Read the model definition and answer for the solid it produces. Units are mm, in the model's axes. Face numbers are marked on the shaded views. A direction names the side the tool comes from. Give positions to 0.01 mm unless a question says otherwise; leave off trailing zeros. Loops run counter-clockwise (first coordinate to the right, second up) from the corner with the lowest first, then second, coordinate; pieces in that order, holes last. Notation, with made-up numbers: (6.5, 49) - (20.5, 49) arc R30 ccw to (20.5, 88) - close; hole circle Ø9 at (55, -20). An arc over 180 degrees is marked (long way). Write each question's results on one line, items separated by ' | '. Start each with the question number.
Q1. The part is cut by section A-A, the plane z = 1. Write down the section's boundary in (x, y).
Q2. The part is cut by section C-C, the plane y = 81.5. Write down the section's boundary in (x, z), plus the area to 3 significant figures.
Q3. Given pin 1 (1.5 mm diameter, centred on x = 3.5, z = 1.5, fed in from -Y); pin 2 (2.5 mm diameter, centred on x = -5, z = 6, fed in from -Y); pin 3 (2.5 mm diameter, centred on x = 0, y = 100, fed in from -Z); pin 4 (2 mm diameter, centred on y = 93.5, z = 4.5, fed in from -X), each flat-ended and moving along its own axis, determine where each tip first touches the part or whether it passes through.
Q4. The part is cut by section D-D, the plane z = 6. State how many separate pieces and enclosed holes the cut face has, plus the area to 3 significant figures.
Q5. For the marked faces 4, 5, 6 and 7, determine the directions among +Z, -Z, +X, -X, +Y, -Y from which every point of the face is accessible in a straight line to the end or side of a thin tool.
Q6. Find the intervals of material crossed by line 1 (Y direction, x = 0, z = 1.6); line 2 (X direction, y = 55.5, z = 6); line 3 (Y direction, x = 11.5, z = 8.5), in increasing order. Write a range as from..to.
Q7. Determine the mould class of the marked faces 1, 2 and 3 for opening direction Y: +Y half, -Y half, draft (parallel to the pull), parting line (faces both ways), or undercut.
Q8. The part is cut by section B-B, the plane x = -8. Write down the section's boundary in (y, z).
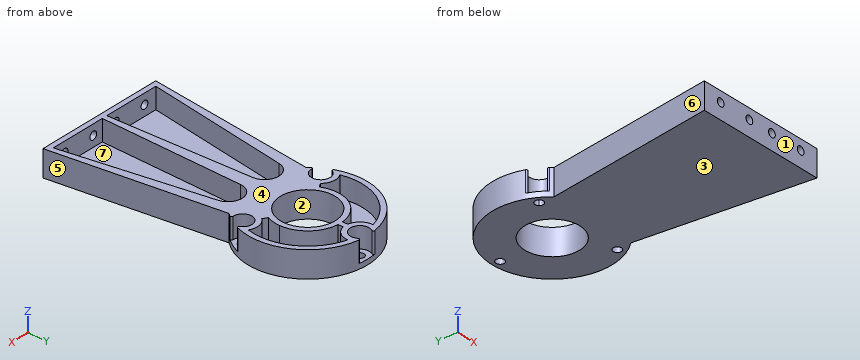
```python
from build123d import *

# Parameters (mm, degrees)
SKETCH_1_R          = 10.5
EXTRUDE_1_DEPTH     = 10
CUT_EXTRUDE_2_DEPTH = 8
SKETCH_3_R          = 1.5
CUT_EXTRUDE_3_DEPTH = 97.81941954
EXTRUDE_START       = -10
SKETCH_4_R          = 1.6
EXTRUDE_3_DEPTH     = 10
CUT_EXTRUDE_START   = -10
SKETCH_5_R          = 1.6
CUT_EXTRUDE_4_DEPTH = 10
CUT_EXTRUDE_START_2 = -8
SKETCH_6_R          = 1.6
CUT_EXTRUDE_5_DEPTH = 8
FILLET_1_R          = 0.5


with BuildPart() as part:
    # 草图1 → 凸台-拉伸1 (new body)
    with BuildSketch(Plane.XY):
        with BuildLine():
            Line((-25, 0), (25, 0))
            Line((25, 0), (14.88676655, 81.839614547))
            ThreePointArc((14.88676655, 81.839614547), (0, 95), (-14.88676655, 81.839614547))
            Line((-14.88676655, 81.839614547), (-25, 0))
        make_face()
        with Locations((0, 80)):
            Circle(SKETCH_1_R, mode=Mode.SUBTRACT)
    extrude(amount=EXTRUDE_1_DEPTH)

    # 草图2 → 切除-拉伸2 (cut)
    with BuildSketch(Plane.XY.offset(10)):
        with BuildLine():
            Line((-13.564970556, 57.262621959), (-22.737639737, 2))
            Line((-22.737639737, 2), (-1, 2))
            Line((-1, 2), (-2.641694958, 56.527552532))
            ThreePointArc((-2.641694958, 56.527552532), (-7.769922801, 61.84962447), (-13.564970556, 57.262621959))
        make_face()
        with BuildLine():
            Line((2.641694958, 56.527552532), (1, 2))
            Line((1, 2), (22.737639737, 2))
            Line((22.737639737, 2), (13.564970556, 57.262621959))
            ThreePointArc((13.564970556, 57.262621959), (7.769922801, 61.84962447), (2.641694958, 56.527552532))
        make_face()
    extrude(amount=-CUT_EXTRUDE_2_DEPTH, mode=Mode.SUBTRACT)

    # 草图3 → 切除-拉伸3 (cut, through all)
    with BuildSketch(Plane(origin=(0, 2, 0), x_dir=(1, 0, 0), z_dir=(0, 1, 0))):
        with Locations(Location((-17.74, -6, 0), (0, 0, 180))):
            Circle(SKETCH_3_R)
        with Locations(Location((-5, -6, 0), (0, 0, 180))):
            Circle(SKETCH_3_R)
        with Locations(Location((5, -6, 0), (0, 0, 180))):
            Circle(SKETCH_3_R)
        with Locations(Location((17.74, -6, 0), (0, 0, 180))):
            Circle(SKETCH_3_R)
    extrude(amount=-CUT_EXTRUDE_3_DEPTH, mode=Mode.SUBTRACT)

    # 草图4 → 凸台-拉伸3 (add)
    with BuildSketch(Plane.XY.offset(10).offset(EXTRUDE_START)):
        with BuildLine():
            Line((16.521104317, 68.614015285), (17.025084925, 64.535638283))
            ThreePointArc((17.025084925, 64.535638283), (0, 103), (-17.025084925, 64.535638283))
            Line((-17.025084925, 64.535638283), (-16.521104317, 68.614015285))
            ThreePointArc((-16.521104317, 68.614015285), (-18.908429841, 70.196225552), (-16.207760954, 71.149692934))
            Line((-16.207760954, 71.149692934), (-14.88676655, 81.839614547))
            ThreePointArc((-14.88676655, 81.839614547), (0, 95), (14.88676655, 81.839614547))
            Line((14.88676655, 81.839614547), (16.207760954, 71.149692934))
            ThreePointArc((16.207760954, 71.149692934), (18.908429841, 70.196225552), (16.521104317, 68.614015285))
        make_face()
        with Locations((0, 100)):
            Circle(SKETCH_4_R, mode=Mode.SUBTRACT)
    extrude(amount=EXTRUDE_3_DEPTH)

    # 草图5 → 切除-拉伸4 (cut)
    with BuildSketch(Plane.XY.offset(10).offset(CUT_EXTRUDE_START)):
        with Locations((-17.320508076, 70)):
            Circle(SKETCH_5_R)
        with Locations((17.320508076, 70)):
            Circle(SKETCH_5_R)
    extrude(amount=CUT_EXTRUDE_4_DEPTH, mode=Mode.SUBTRACT)

    # 草图6 → 切除-拉伸5 (cut)
    # profile 1 of 5: a face of its own
    with BuildSketch(Plane.XY.offset(10).offset(CUT_EXTRUDE_START_2)):
        with BuildLine():
            ThreePointArc((-13.04871596, 73.621020867), (-16.480843406, 75.536692446), (-20.326626095, 74.724749142))
            ThreePointArc((-20.326626095, 74.724749142), (-18.186533479, 90.5), (-5.594811793, 100.241))
            ThreePointArc((-5.594811793, 100.241), (-4.375083977, 96.504482843), (-1, 94.490009074))
            Line((-1, 94.490009074), (-1, 92.459935794))
            ThreePointArc((-1, 92.459935794), (-10.825317547, 86.25), (-11.290620927, 74.636057507))
            Line((-11.290620927, 74.636057507), (-13.04871596, 73.621020867))
        make_face()
    # profile 2 of 5: a face of its own
    with BuildSketch(Plane.XY.offset(10).offset(CUT_EXTRUDE_START_2)):
        with BuildLine():
            ThreePointArc((2.131712692, 102.901), (0, 103), (-2.131712692, 102.901))
            ThreePointArc((-2.131712692, 102.901), (-1.625705125, 96.787978387), (3.6, 100))
            ThreePointArc((3.6, 100), (3.212021613, 101.625705125), (2.131712692, 102.901))
        make_face()
        with Locations((0, 100)):
            Circle(SKETCH_6_R, mode=Mode.SUBTRACT)
    # profile 3 of 5: a face of its own
    with BuildSketch(Plane.XY.offset(10).offset(CUT_EXTRUDE_START_2)):
        with BuildLine():
            ThreePointArc((12.5, 80), (12.193907528, 77.25070569), (11.290620927, 74.636057507))
            Line((11.290620927, 74.636057507), (13.04871596, 73.621020867))
            ThreePointArc((13.04871596, 73.621020867), (16.480843406, 75.536692446), (20.326626095, 74.724749142))
            ThreePointArc((20.326626095, 74.724749142), (18.186533479, 90.5), (5.594811793, 100.241))
            ThreePointArc((5.594811793, 100.241), (4.375083977, 96.504482843), (1, 94.490009074))
            Line((1, 94.490009074), (1, 92.459935794))
            ThreePointArc((1, 92.459935794), (9.185586535, 88.477912479), (12.5, 80))
        make_face()
    # profile 4 of 5: a face of its own
    with BuildSketch(Plane.XY.offset(10).offset(CUT_EXTRUDE_START_2)):
        with BuildLine():
            ThreePointArc((18.766991426, 66.703382655), (19.918584287, 68.5), (20.898704118, 70.395617345))
            ThreePointArc((20.898704118, 70.395617345), (14.202816622, 71.8), (18.766991426, 66.703382655))
        make_face()
        with BuildLine():
            ThreePointArc((16.207760954, 71.149692934), (17.944849571, 71.473159088), (18.920508076, 70))
            ThreePointArc((18.920508076, 70), (18.120806141, 68.614531485), (16.521104317, 68.614015285))
            ThreePointArc((16.521104317, 68.614015285), (15.73258631, 69.803774448), (16.207760954, 71.149692934))
        make_face(mode=Mode.SUBTRACT)
    # profile 5 of 5: a face of its own
    with BuildSketch(Plane.XY.offset(10).offset(CUT_EXTRUDE_START_2)):
        with BuildLine():
            ThreePointArc((-18.766991426, 66.703382655), (-15.351668324, 66.986087256), (-13.720508076, 70))
            ThreePointArc((-13.720508076, 70), (-17.122399207, 73.594544877), (-20.898704118, 70.395617345))
            ThreePointArc((-20.898704118, 70.395617345), (-19.918584287, 68.5), (-18.766991426, 66.703382655))
        make_face()
        with Locations((-17.320508076, 70)):
            Circle(SKETCH_6_R, mode=Mode.SUBTRACT)
    extrude(amount=CUT_EXTRUDE_5_DEPTH, mode=Mode.SUBTRACT)

    # 圆角1
    fillet_1_edges = [part.edges().sort_by_distance(p)[0] for p in [
        (-2.131712692, 102.901, 6),
        (2.131712692, 102.901, 6),
        (20.898704118, 70.395617345, 6),
        (18.766991426, 66.703382655, 6),
        (-18.766991426, 66.703382655, 6),
        (-20.898704118, 70.395617345, 6),
    ]]
    fillet(fillet_1_edges, radius=FILLET_1_R)


solid = part.part
```
Check sheet entries:
1) outline: (-25, 0) - (25, 0) - (17.03, 64.54) arc R23 ccw (long way) to (-17.03, 64.54) - close; hole circle Ø3.2 at (-17.32, 70); hole circle Ø21 at (0, 80); hole circle Ø3.2 at (0, 100); hole circle Ø3.2 at (17.32, 70)
2) outline: (-22.95, 0) - (-10.39, 0) - (-10.39, 10) - (-12.41, 10) - (-12.41, 2) - (-20.95, 2) - (-20.95, 10) - (-22.95, 10) - close; (10.39, 0) - (22.95, 0) - (22.95, 10) - (20.95, 10) - (20.95, 2) - (12.41, 2) - (12.41, 10) - (10.39, 10) - close | area: 115 mm^2
3) pin 1: stops at y = 0 | pin 2: stops at y = 59.68 | pin 3: passes through | pin 4: stops at x = -19.31
4) separate pieces: 3 | enclosed holes: 3 | area: 1,350 mm^2
5) face 4: +Z, +X, -X, +Y, -Y | face 5: +Z, -Z, +X | face 6: +Z, -Z, -X | face 7: +Z
6) line 1: y = 0..69.5, 90.5..98.4, 101.6..103 | line 2: x = -18.14..-13.86, -2.61..2.61, 13.86..18.14 | line 3: y = 0..2, 60.72..74.52, 75.1..84.9, 97.57..99.92
7) face 1: -Y half | face 2: undercut | face 3: draft
8) outline: (0, 0) - (73.2, 0) - (73.2, 10) - (61.86, 10) - (61.86, 2) - (2, 2) - (2, 10) - (0, 10) - close; (86.8, 0) - (101.56, 0) - (101.56, 10) - (99.42, 10) - (99.42, 2) - (89.6, 2) - (89.6, 10) - (86.8, 10) - close
